```python
from build123d import *

# Parameters (mm, degrees)
SKETCH1_R                = 3
SKETCH1_W                = 18.5
SKETCH1_H                = 30
BOSS_EXTRUDE1_DEPTH      = 18.28
CUT_EXTRUDE1_START       = -32.5
CUT_EXTRUDE1_OUTLINE_R   = 3.75
CUT_EXTRUDE1_OUTLINE_R_2 = 2.55
CUT_EXTRUDE1_DEPTH       = 32.5
CUT_EXTRUDE2_DEPTH       = 3
SKETCH4_W                = 4.2
SKETCH4_H                = 8.5
CUT_EXTRUDE3_DEPTH       = 11.67582
CUT_EXTRUDE4_DEPTH       = 2


# Read off the part's stored shape, not the designer's step: Cut-Extrude1
with BuildPart() as part:
    # Sketch1 → Boss-Extrude1 (new body)
    with BuildSketch(Plane(origin=(0, 0, 0), x_dir=(1, 0, 0), z_dir=(0, 1, 0))):
        with BuildLine():
            Line((0, 0), (32.5, 0))
            Line((32.5, 0), (32.5, 65))
            ThreePointArc((32.5, 65), (31.035533906, 68.535533906), (27.5, 70))
            Line((27.5, 70), (20.403311931, 70))
            ThreePointArc((20.403311931, 70), (16.25, 71.5), (12.096688069, 70))
            Line((12.096688069, 70), (5, 70))
            ThreePointArc((5, 70), (1.464466094, 68.535533906), (0, 65))
            Line((0, 65), (0, 0))
        make_face()
        with Locations(Location((16.25, 65, 0), (0, 0, 270))):
            Circle(SKETCH1_R, mode=Mode.SUBTRACT)
        with Locations((16.25, 35)):
            Rectangle(SKETCH1_W, SKETCH1_H, mode=Mode.SUBTRACT)
    extrude(amount=BOSS_EXTRUDE1_DEPTH)

    # Cut-Extrude1 outline → Cut-Extrude1 (cut)
    with BuildSketch(Plane.ZY.offset(CUT_EXTRUDE1_START)):
        with BuildLine():
            Line((-73, 5), (-52.220306773, 5))
            ThreePointArc((-52.220306773, 5), (-46.908361498, 6.734792681), (-43.644221508, 11.270391691))
            ThreePointArc((-43.644221508, 11.270391691), (-34.353354825, 17.615612411), (-25.952469379, 10.131819693))
            ThreePointArc((-25.952469379, 10.131819693), (-20.659340598, 5.058687621), (-14.189782649, 8.508137035))
            ThreePointArc((-14.189782649, 8.508137035), (-11.238803116, 11.78472904), (-7, 13))
            Line((-7, 13), (-5, 13))
            ThreePointArc((-5, 13), (-1.464466094, 11.535533906), (0, 8))
            Line((0, 8), (0, 18.28))
            Line((0, 18.28), (-73, 18.28))
            Line((-73, 18.28), (-73, 5))
        make_face()
        with BuildLine():
            Line((-5, 0), (-20, 1e-09))
            Line((-20, 1e-09), (-20, -1))
            Line((-20, -1), (0, -1))
            Line((0, -1), (0, 5))
            ThreePointArc((0, 5), (-1.464466094, 1.464466094), (-5, 0))
        make_face()
        with Locations((-34.94, 8.5)):
            Circle(CUT_EXTRUDE1_OUTLINE_R)
        with Locations((-6, 6.5)):
            Circle(CUT_EXTRUDE1_OUTLINE_R_2)
    extrude(amount=CUT_EXTRUDE1_DEPTH, mode=Mode.SUBTRACT)

    # Sketch3 → Cut-Extrude2 (cut)
    with BuildSketch(Plane.ZY):
        Polygon((-26.857096231, 8.5), (-30.898548116, 15.5), (-38.981451884, 15.5), (-43.022903769, 8.5), (-38.981451884, 1.5), (-30.898548116, 1.5), align=None)
    cut_extrude2 = extrude(amount=-CUT_EXTRUDE2_DEPTH, mode=Mode.SUBTRACT)

    # Mirror1: Cut-Extrude2 across plane
    add(cut_extrude2.mirror(Plane.ZY.offset(-16.25)), mode=Mode.SUBTRACT)

    # Sketch4 → Cut-Extrude3 (cut)
    with BuildSketch(Plane.XY):
        with Locations((5.55, 6.5)):
            Rectangle(SKETCH4_W, SKETCH4_H)
    cut_extrude3 = extrude(amount=-CUT_EXTRUDE3_DEPTH, mode=Mode.SUBTRACT)

    # Mirror2: Cut-Extrude3 across plane
    add(cut_extrude3.mirror(Plane.ZY.offset(-16.25)), mode=Mode.SUBTRACT)

    # Sketch5 → Cut-Extrude4 (cut)
    with BuildSketch(Plane.XZ):
        Polygon((11.515727793, -65), (13.882863896, -69.1), (18.617136104, -69.1), (20.984272207, -65), (18.617136104, -60.9), (13.882863896, -60.9), align=None)
    extrude(amount=-CUT_EXTRUDE4_DEPTH, mode=Mode.SUBTRACT)


solid = part.part
```
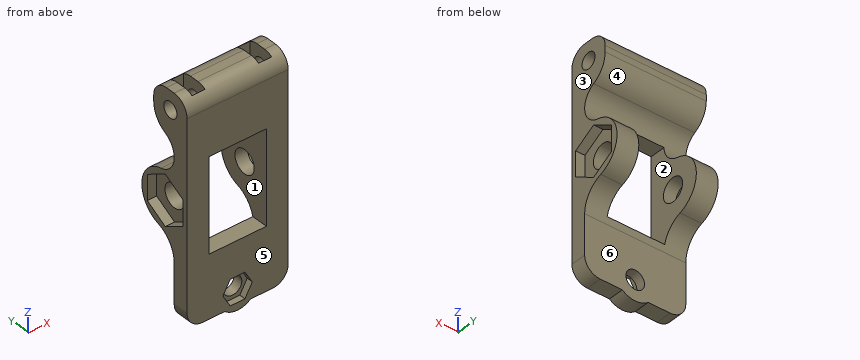
Read the model definition and answer for the solid it produces. Units are mm, in the model's axes. Face numbers are marked on the shaded views. A direction names the side the tool comes from. Round coordinates to 2 decimals unless told otherwise and drop trailing zeros. Write each loop counter-clockwise with the first axis right and the second up, starting at its lowest first coordinate (ties: lowest second). Pieces come first, ordered by that corner, then holes. Notation, with made-up numbers: (44, -4.5) -> (93, -4.5) arc R6 ccw to (93, 3.5) -> close; hole circle Ø2 at (-30.5, 66). An arc over 180 degrees is marked (long way). Answer in a Markdown table with one row per item. Add a question column.
1) Find section D-D, the plane z = -6. Determine the outline of the cut face in (x, y), and give its area (3 significant figures).
2) Find section B-B, the plane x = 16.25. Determine the outline of the cut face in (y, z) (3 decimals).
3) Given P1, Ø6, axis at y = 8.5, z = -34.94, coming from the -X side; P2, Ø1.6, axis at x = 15, y = 1.5, coming from the -Z side; P3, Ø1.5, axis at x = 25.5, y = 3, coming from the -Z side; P4, Ø4, axis at x = 24.5, y = 15.5, coming from the +Z side, each flat-ended and moving along its own axis, determine where each tip first touches the part or whether it passes through.
4) Determine the mould class of the marked faces 1, 2, 3 and 4 for opening direction X: pulls with the +X half, pulls with the -X half, needs draft (parallel to the pull), parting line crosses it, or undercut.
5) Find section A-A, the plane x = 23.5. Determine the outline of the cut face in (y, z) (3 decimals).
6) Consider line 1 (X direction, y = 2.5, z = -5); line 2 (Y direction, x = 30.3, z = -6); line 3 (X direction, y = 4.1, z = -65). Determine where each line is inside the solid, lowest interval first.
7) Which of the six approach directions +Z, -Z, +X, -X, +Y, -Y give full straight-line access (tool end or side, diameter ignored) to the marked faces 5 and 6?
8) Find section C-C, the plane z = -34.94. Determine the outline of the cut face in (x, y), and give its area (3 significant figures).
Findings below:
| question | item | result |
|---|---|---|
| 1 | outline | (0, 0) -> (32.5, 0) -> (32.5, 3.95) -> (29.05, 3.95) -> (29.05, 2.25) -> (24.85, 2.25) -> (24.85, 3.95) -> (7.65, 3.95) -> (7.65, 2.25) -> (3.45, 2.25) -> (3.45, 3.95) -> (0, 3.95) -> close; (0, 9.05) -> (3.45, 9.05) -> (3.45, 10.75) -> (7.65, 10.75) -> (7.65, 9.05) -> (24.85, 9.05) -> (24.85, 10.75) -> (29.05, 10.75) -> (29.05, 9.05) -> (32.5, 9.05) -> (32.5, 13) -> (0, 13) -> close |
| 1 | area | 228 mm² |
| 2 | outline | (0, -71.5) -> (5, -71.5) -> (5, -68) -> (2, -68) -> (2, -69.1) -> (0, -69.1) -> close; (0, -60.9) -> (2, -60.9) -> (2, -62) -> (5, -62) -> (5, -52.22) arc R9 cw to (5.278, -50) -> (0, -50) -> close; (0, -20) -> (5.003, -20) arc R6.248 cw to (8.508, -14.19) arc R8 ccw to (13, -7) -> (13, -5) arc R5 ccw to (8, 0) -> (5, 0) arc R5 ccw to (0, -5) -> close; hole circle Ø5.1 at (6.5, -6) |
| 3 | P1 | through |
| 3 | P2 | z = -71.48 |
| 3 | P3 | z = -70 |
| 3 | P4 | z = -27.48 |
| 4 | face 1 | undercut |
| 4 | face 2 | undercut |
| 4 | face 3 | pulls with the +X half |
| 4 | face 4 | needs draft |
| 5 | outline | (0, -70) -> (5, -70) -> (5, -52.22) arc R9 cw to (5.278, -50) -> (0, -50) -> close; (0, -20) -> (5.003, -20) arc R6.248 cw to (8.508, -14.19) arc R8 ccw to (13, -7) -> (13, -5) arc R5 ccw to (8, 0) -> (5, 0) arc R5 ccw to (0, -5) -> close; hole circle Ø5.1 at (6.5, -6) |
| 6 | line 1 | 0 to 3.45, 7.65 to 24.85, 29.05 to 32.5 |
| 6 | line 2 | 0 to 3.95, 9.05 to 13 |
| 6 | line 3 | 0 to 13.25, 19.25 to 32.5 |
| 7 | face 5 | +Z, -Z, +X, -X, -Y |
| 7 | face 6 | -Z, +X, -X, +Y |
| 8 | outline | (0, 0) -> (7, 0) -> (7, 4.75) -> (3, 4.75) -> (3, 1.5) -> (0, 1.5) -> close; (0, 15.5) -> (3, 15.5) -> (3, 12.25) -> (7, 12.25) -> (7, 17.63) -> (0, 17.63) -> close; (25.5, 0) -> (32.5, 0) -> (32.5, 1.5) -> (29.5, 1.5) -> (29.5, 4.75) -> (25.5, 4.75) -> close; (25.5, 12.25) -> (29.5, 12.25) -> (29.5, 15.5) -> (32.5, 15.5) -> (32.5, 17.63) -> (25.5, 17.63) -> close |
| 8 | area | 103 mm² |
